from build123d import *

# Parameters (mm, degrees)
SKETCH_1_W      = 300
SKETCH_1_H      = 150
EXTRUDE_1_DEPTH = 10
SKETCH_2_R      = 10
EXTRUDE_2_DEPTH = 40
FILLET_1_R      = 4


with BuildPart() as part:
    # 草圖1 → 填料-伸長1 (new body)
    with BuildSketch(Plane.XY):
        with Locations((150, 75)):
            Rectangle(SKETCH_1_W, SKETCH_1_H)
    extrude(amount=EXTRUDE_1_DEPTH)

    # 草圖2 → 填料-伸長2 (add)
    with BuildSketch(Plane.XY.offset(10)):
        with Locations(Location((90, 75, 0), (0, 0, 180))):
            Circle(SKETCH_2_R)
        with Locations(Location((210, 75, 0), (0, 0, 180))):
            Circle(SKETCH_2_R)
    extrude(amount=EXTRUDE_2_DEPTH)

    # 圓角1
    fillet_1_edges = [part.edges().sort_by_distance(p)[0] for p in [
        (300, 75, 10),
        (150, 150, 10),
        (100, 75, 10),
        (100, 75, 50),
        (220, 75, 10),
        (220, 75, 50),
        (0, 75, 10),
        (150, 150, 0),
        (300, 75, 0),
        (150, 0, 0),
        (0, 75, 0),
        (150, 0, 10),
        (0, 150, 5),
        (300, 150, 5),
        (300, 0, 5),
        (0, 0, 5),
    ]]
    fillet(fillet_1_edges, radius=FILLET_1_R)


solid = part.part
Build history of the part. All positions in model axes, mm. A direction names the side the tool comes from. Round coordinates to 2 decimals unless told otherwise and drop trailing zeros. Write each loop counter-clockwise with the first axis right and the second up, starting at its lowest first coordinate (ties: lowest second). Pieces come first, ordered by that corner, then holes. Notation, with made-up numbers: M -30.75,29 L 23.25,29 A18 ccw 23.25,49 Z; hole C 29,-16 d9. An arc over 180 degrees is marked long. Answer as a JSON object with one key per item and string values. Group by question number.
(1) Flat gauge pins, fed straight in: pin 1 (6 mm diameter, centred on y = 80, z = 19.5, fed in from -X); pin 2 (6 mm diameter, centred on y = 75, z = 12, fed in from +X); pin 3 (5 mm diameter, centred on x = 250.5, y = 77, fed in from +Z). Where does each tip first touch, or does it go through?
(2) Drill centre lines: L1, parallel to Z at x = 230, y = 56.5; L2, parallel to X at y = 75.5, z = 46; L3, parallel to X at y = 68.5, z = 22. Where is each one in solid material? Low to high.
(3) Cut at D-D (x = 161). Give the cut face in (y, z), and give its area (3 significant figures).
(4) Cut at A-A (y = 75). Give the cut face in (x, z), and give its area (3 significant figures).
(5) Mould opens along X. For faces 1 (the flat face through (90, 75, 50)), 2 (the cylindrical face through (200.46, 72, 29.78)) say: pulls with the +X half, pulls with the -X half, needs draft (parallel to the pull), parting line crosses it, or undercut.
(6) Cut at B-B (x = 90). Give the cut face in (y, z).
(7) Cut at C-C (z = 21.5). Give the cut face in (x, y), and give its area (3 significant figures).
(8) Which spindle directions (+Z, -Z, +X, -X, +Y, -Y) get a long thin tool onto all of the face, cutting with end or side? Do faces 3 (the flat face through (148, 76, 0)), 4 (the cylindrical face through (100, 75, 30)). Say none if no direction does.
Responses:
{
 "1": {"pin 1": "stops at x = 80.2", "pin 2": "stops at x = 298.65", "pin 3": "stops at z = 10"},
 "2": {"L1": "z = 0 to 10", "L2": "x = 80.01 to 99.99, 200.01 to 219.99", "L3": "x = 82.4 to 97.6, 202.4 to 217.6"},
 "3": {"outline": "M 0,4 A4 ccw 4,0 L 146,0 A4 ccw 150,4 L 150,6 A4 ccw 146,10 L 4,10 A4 ccw 0,6 Z", "area": "1,490 mm2"},
 "4": {"outline": "M 0,4 A4 ccw 4,0 L 296,0 A4 ccw 300,4 L 300,6 A4 ccw 296,10 L 224,10 A4 cw 220,14 L 220,46 A4 ccw 216,50 L 204,50 A4 ccw 200,46 L 200,14 A4 cw 196,10 L 104,10 A4 cw 100,14 L 100,46 A4 ccw 96,50 L 84,50 A4 ccw 80,46 L 80,14 A4 cw 76,10 L 4,10 A4 ccw 0,6 Z", "area": "4,590 mm2"},
 "5": {"face 1": "needs draft", "face 2": "undercut"},
 "6": {"outline": "M 0,4 A4 ccw 4,0 L 146,0 A4 ccw 150,4 L 150,6 A4 ccw 146,10 L 89,10 A4 cw 85,14 L 85,46 A4 ccw 81,50 L 69,50 A4 ccw 65,46 L 65,14 A4 cw 61,10 L 4,10 A4 ccw 0,6 Z"},
 "7": {"outline": "C 90,75 d20; C 210,75 d20", "area": "628 mm2"},
 "8": {"face 3": "-Z, +X, -X, +Y, -Y", "face 4": "+Z"}
}
